CAD build for the part. Positions are in the model's coordinates, mm. Face numbers are marked on the shaded views. A direction names the side the tool comes from. Round coordinates to 2 decimals unless told otherwise and drop trailing zeros. Write each loop counter-clockwise with the first axis right and the second up, starting at its lowest first coordinate (ties: lowest second). Pieces come first, ordered by that corner, then holes. Notation, with made-up numbers: (-14, 88.5) -> (19, 88.5) arc R30 ccw to (19, 114.5) -> close; hole circle Ø1 at (33, 83.5). An arc over 180 degrees is marked (long way). Put each result on its own line as item: value. Start each with the question number.
1. Drill centre lines: line 1 (Z direction, x = 0, y = 3.6); line 2 (Z direction, x = 0, y = 0.65); line 3 (X direction, y = -1.15, z = -0.5). Where is each one in solid material? Low to high. Write a range as from..to.
2. Pull direction X, two halves, no side cores. Call the marked faces 1, 2 and 3: pulls with the +X half, pulls with the -X half, needs draft (parallel to the pull), parting line crosses it, or undercut.
3. Saw through at A-A on y = 1.2. List the corners of the cut face in (x, z).
4. 3-axis set-ups, long thin cutter, end or side, ignore diameter. For the marked faces 4 and 5: which of +Z, -Z, +X, -X, +Y, -Y reach the whole face in a straight line?
5. Flat gauge pins, fed straight in: P1, Ø3, axis at x = -1.5, z = -13, coming from the -Y side; P2, Ø15.5, axis at x = -3.5, z = 3, coming from the +Y side (1 decimal); P3, Ø1.5, axis at y = -1, z = 13.5, coming from the +X side; P4, Ø1.5, axis at x = -15, y = 0, coming from the -Z side. Where does each tip first touch, or does it go through?
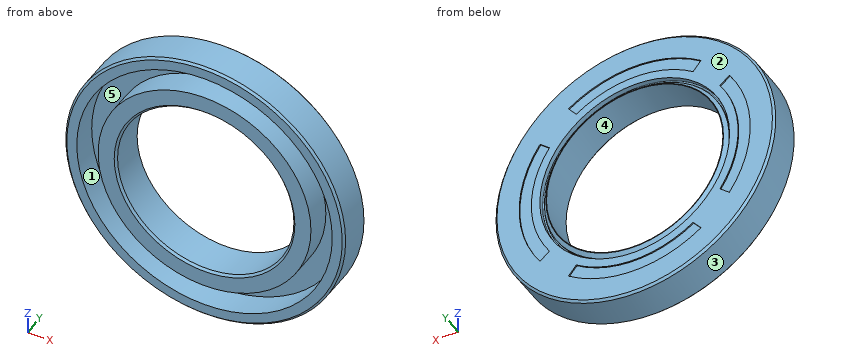
from build123d import *

# Parameters (mm, degrees)
CUT_EXTRUDE1_DEPTH = 0.2
CIRPATTERN1_COUNT  = 4


with BuildPart() as part:
    # Sketch1 → Revolve1 (revolve)
    with BuildSketch(Plane.XY):
        with BuildLine():
            ThreePointArc((15.4, 3.241206918), (15.541421356, 3.299785562), (15.6, 3.441206918))
            Line((15.6, 3.441206918), (15.6, 4.241206918))
            Line((15.6, 4.241206918), (22.646446609, 4.241206918))
            Line((22.646446609, 4.241206918), (23, 3.887653527))
            Line((23, 3.887653527), (23, -1.405239692))
            Line((23, -1.405239692), (22.646446609, -1.758793082))
            Line((22.646446609, -1.758793082), (21, -1.758793082))
            Line((21, -1.758793082), (21, 2.541206918))
            Line((21, 2.541206918), (17.5, 2.541206918))
            Line((17.5, 2.541206918), (17.5, -1.758793082))
            Line((17.5, -1.758793082), (14.853553391, -1.758793082))
            Line((14.853553391, -1.758793082), (14.5, -1.405239692))
            Line((14.5, -1.405239692), (14.5, 3.887653527))
            Line((14.5, 3.887653527), (14.5, 4.241206918))
            Line((14.5, 4.241206918), (14.6, 4.241206918))
            Line((14.6, 4.241206918), (15.2, 3.641206918))
            Line((15.2, 3.641206918), (15.2, 3.241206918))
            Line((15.2, 3.241206918), (15.4, 3.241206918))
        make_face()
    revolve(axis=Axis((0, 10.772096588, 0), (0, -1, 0)))

    # Sketch2 → Cut-Extrude1 (cut)
    with BuildSketch(Plane(origin=(0, 4.241206918, 0), x_dir=(1, 0, 0), z_dir=(0, 1, 0))):
        with BuildLine():
            Line((-14.025254522, -9.606884801), (-15.563888841, -10.897952291))
            ThreePointArc((-15.563888841, -10.897952291), (-19, 0), (-15.563888841, 10.897952291))
            Line((-15.563888841, 10.897952291), (-14.025254522, 9.606884801))
            ThreePointArc((-14.025254522, 9.606884801), (-17, 0), (-14.025254522, -9.606884801))
        make_face()
    cut_extrude1 = extrude(amount=-CUT_EXTRUDE1_DEPTH, mode=Mode.SUBTRACT)

    # CirPattern1: Cut-Extrude1 ×4 about axis
    cirpattern1_axis = Axis((0, 0, 0), (0, 1, 0))
    for i in range(1, CIRPATTERN1_COUNT):
        add(cut_extrude1.rotate(cirpattern1_axis, i * 360 / CIRPATTERN1_COUNT), mode=Mode.SUBTRACT)


solid = part.part
Return value:
1. line 1: z = -23..-15.6, -15.2..-14.5, 14.5..15.2, 15.6..23
1. line 2: z = -23..-21, -17.5..-14.5, 14.5..17.5, 21..23
1. line 3: x = -22.99..-20.99, -17.49..-14.49, 14.49..17.49, 20.99..22.99
2. face 1: undercut
2. face 2: needs draft
2. face 3: parting line crosses it
3. outline: circle Ø46 at (0, 0); circle Ø35 at (0, 0); hole circle Ø42 at (0, 0); hole circle Ø29 at (0, 0)
4. face 4: +Y, -Y
4. face 5: -Y
5. P1: stops at y = -1.49
5. P2: passes through
5. P3: stops at x = 19.14
5. P4: stops at z = -18.05
